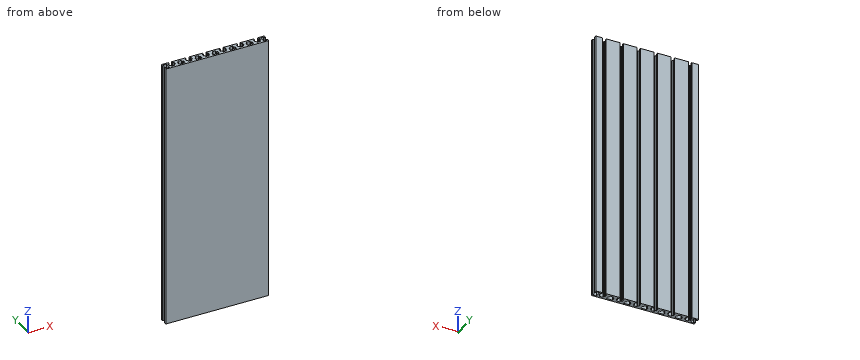
```python
from build123d import *

# Parameters (mm, degrees)
BOSS_EXTRUDE1_DEPTH = 625


with BuildPart() as part:
    # Sketch1 → Boss-Extrude1 (new body)
    with BuildSketch(Plane.XY):
        Polygon((-120, 10), (-120, 4.166666667), (-116.945068586, 4.166666667), (-116.945068586, 7.166666667), (-109.945068586, 7.166666667), (-109.945068586, -7.166666667), (-116.945068586, -7.166666667), (-116.945068586, -4.166666667), (-120, -4.166666667), (-120, -10), (120, -10), (120, -4.166666667), (116.945068586, -4.166666667), (116.945068586, -7.166666667), (109.945068586, -7.166666667), (109.945068586, 7.166666667), (116.945068586, 7.166666667), (116.945068586, 4.166666667), (120, 4.166666667), (120, 10), (104.166666667, 10), (104.166666667, 6), (107.166666667, 6), (107.166666667, -1), (104.166666667, -1), (104.166666667, -5.093909387), (95.833333333, -5.093909387), (95.833333333, -1), (92.833333333, -1), (92.833333333, 6), (95.833333333, 6), (95.833333333, 10), (64.166666667, 10), (64.166666667, 6), (67.166666667, 6), (67.166666667, -1), (64.166666667, -1), (64.166666667, -5.093909387), (55.833333333, -5.093909387), (55.833333333, -1), (52.833333333, -1), (52.833333333, 6), (55.833333333, 6), (55.833333333, 10), (24.166666667, 10), (24.166666667, 6), (27.166666667, 6), (27.166666667, -1), (24.166666667, -1), (24.166666667, -5.093909387), (15.833333333, -5.093909387), (15.833333333, -1), (12.833333333, -1), (12.833333333, 6), (15.833333333, 6), (15.833333333, 10), (-15.833333333, 10), (-15.833333333, 6), (-12.833333333, 6), (-12.833333333, -1), (-15.833333333, -1), (-15.833333333, -5.093909387), (-24.166666667, -5.093909387), (-24.166666667, -1), (-27.166666667, -1), (-27.166666667, 6), (-24.166666667, 6), (-24.166666667, 10), (-55.833333333, 10), (-55.833333333, 6), (-52.833333333, 6), (-52.833333333, -1), (-55.833333333, -1), (-55.833333333, -5.093909387), (-64.166666667, -5.093909387), (-64.166666667, -1), (-67.166666667, -1), (-67.166666667, 6), (-64.166666667, 6), (-64.166666667, 10), (-95.833333333, 10), (-95.833333333, 6), (-92.833333333, 6), (-92.833333333, -1), (-95.833333333, -1), (-95.833333333, -5.093909387), (-104.166666667, -5.093909387), (-104.166666667, -1), (-107.166666667, -1), (-107.166666667, 6), (-104.166666667, 6), (-104.166666667, 10), align=None)
        Polygon((-72.833333333, -6), (-87.166666667, -6), (-87.166666667, 1), (-84.166666667, 1), (-84.166666667, 5.362249924), (-75.833333333, 5.362249924), (-75.833333333, 1), (-72.833333333, 1), align=None, mode=Mode.SUBTRACT)
        Polygon((-32.833333333, -6), (-47.166666667, -6), (-47.166666667, 1), (-44.166666667, 1), (-44.166666667, 5.362249924), (-35.833333333, 5.362249924), (-35.833333333, 1), (-32.833333333, 1), align=None, mode=Mode.SUBTRACT)
        Polygon((7.166666667, -6), (-7.166666667, -6), (-7.166666667, 1), (-4.166666667, 1), (-4.166666667, 5.362249924), (4.166666667, 5.362249924), (4.166666667, 1), (7.166666667, 1), align=None, mode=Mode.SUBTRACT)
        Polygon((47.166666667, -6), (32.833333333, -6), (32.833333333, 1), (35.833333333, 1), (35.833333333, 5.362249924), (44.166666667, 5.362249924), (44.166666667, 1), (47.166666667, 1), align=None, mode=Mode.SUBTRACT)
        Polygon((87.166666667, -6), (72.833333333, -6), (72.833333333, 1), (75.833333333, 1), (75.833333333, 5.362249924), (84.166666667, 5.362249924), (84.166666667, 1), (87.166666667, 1), align=None, mode=Mode.SUBTRACT)
    extrude(amount=BOSS_EXTRUDE1_DEPTH)


solid = part.part
```
Verification items for the finished model (mm, model axes). Round coordinates to 2 decimals unless told otherwise and drop trailing zeros.
1. Scan lines: L1, parallel to Y at x = 75.5, z = 305; L2, parallel to Y at x = -54, z = 337; L3, parallel to Y at x = 22, z = 594.5. Record each from-to range of solid material in increasing order.
2. Section check A-A on z = 39.5. State how many separate pieces and enclosed holes the cut face has, plus the area to 3 significant figures.
3. Gauge pin test, flat ends, axial feed: P1, Ø1.5, axis at x = 46, y = 5.5, coming from the -Z side; P2, Ø1.2, axis at y = -2, z = 319.5, coming from the -X side. Record the tip position at first contact, or that the pin passes through.
Answer:
1. L1: y = -10 to -6, 1 to 10
1. L2: y = -10 to -1, 6 to 10
1. L3: y = -10 to -5.09
2. separate pieces: 1
2. enclosed holes: 5
2. area: 2,860 mm2
3. P1: stops at z = 0
3. P2: stops at x = -109.95
